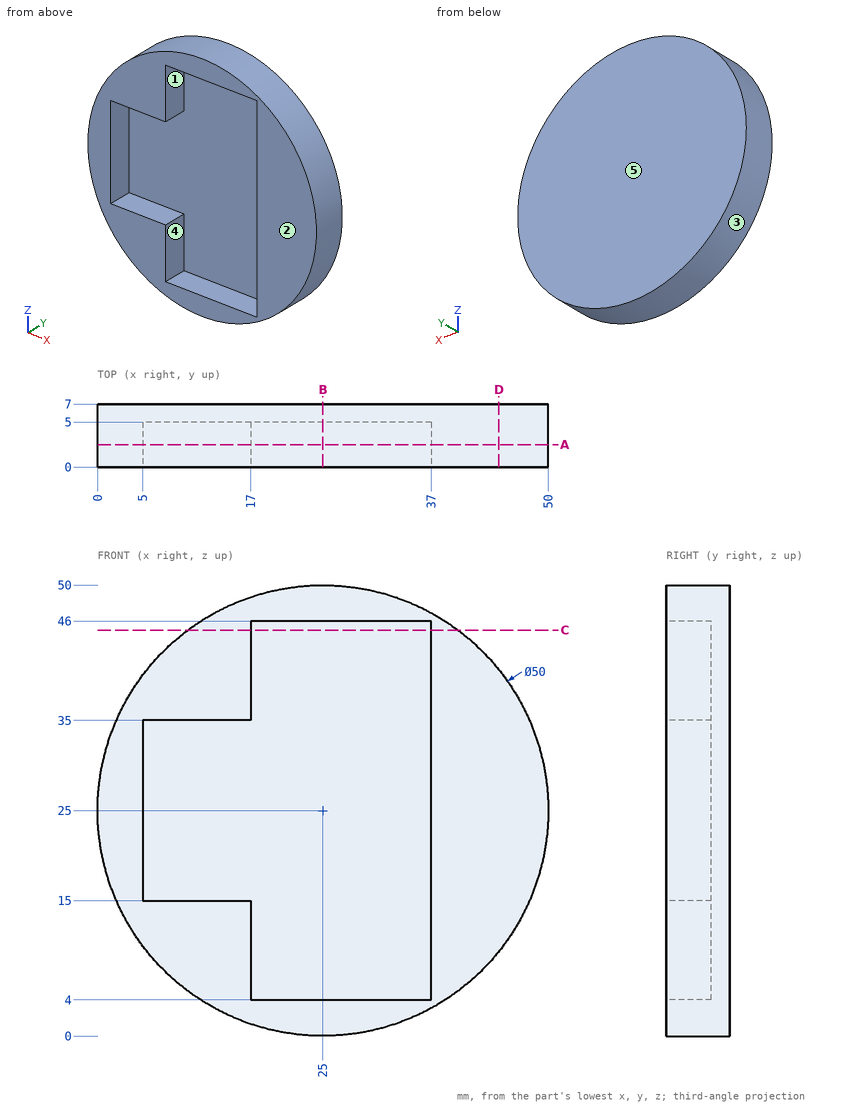
Here's the drawing with two shaded views (mm, measured from the low corner). I have some questions. A direction names the side the tool comes from. Give positions to 0.01 mm unless a question says otherwise; leave off trailing zeros. Order: outer loops, then holes, each group sorted by start corner. A loop starts at its lowest first (then second) coordinate and runs counter-clockwise, first axis right, second up. Notation, with made-up numbers: (-16.5, 11.5) - (37.5, 11.5) arc R16 cw to (37.5, 30.5) - close; hole circle Ø9 at (46, 17.5). An arc over 180 degrees is marked (long way). Write each question's results on one line, items separated by ' | '.
1) Suppose I cut it at D-D, the plane x = 44.5. Write out the boundary of the cut face in (y, z), then the cut area to 3 significant figures.
Final values:
outline: (0, 9.36) - (7, 9.36) - (7, 40.64) - (0, 40.64) - close | area: 219 mm^2
2) Suppose I cut it at C-C, the plane z = 45. Write out the boundary of the cut face in (x, y).
Final values:
outline: (10, 0) - (17, 0) - (17, 5) - (37, 5) - (37, 0) - (40, 0) - (40, 7) - (10, 7) - close
3) If we mould it in two halves opening along Z, with no side actions, what happens to the marked faces 3, 4 and 5? For each: pulls with the +Z half, pulls with the -Z half, needs draft (parallel to the pull), parting line crosses it, or undercut.
Final values:
face 3: parting line crosses it | face 4: undercut | face 5: needs draft
4) Please list where these lines run through material, in increasing order: line 1 along Y through (x, z) = (6.5, 30); line 2 along Z through (x, y) = (33.5, 1); line 3 along X through (y, z) = (3.25, 14). Write a range as [from, to].
Final values:
line 1: y = [5, 7] | line 2: z = [1.49, 4], [46, 48.51] | line 3: x = [2.55, 17], [37, 47.45]
5) I'm going to push flat-ended pins straight in: pin 1 Ø4 at (x, y) = (12, 2.5) entering from +Z; pin 2 Ø1.5 at (x, z) = (40.5, 14) entering from -Y; pin 3 Ø4 at (x, y) = (7.5, 5.5) entering from +Z; pin 4 Ø4 at (y, z) = (1.5, 15.5) entering from -X. Where does each tip first touch, or does it pass through?
Final values:
pin 1: stops at z = 47.45 | pin 2: stops at y = 0 | pin 3: stops at z = 44.62 | pin 4: stops at x = 1.15
6) On a 3-axis mill with a long thin cutter (end or side, diameter ignored), from which of +Z, -Z, +X, -X, +Y, -Y can I reach the whole of each face in a straight line? I mean the marked faces 1 and 2. Say none if no direction works.
Final values:
face 1: -Y | face 2: +Z, -Z, +X, -X, -Y
7) Suppose I cut it at B-B, the plane x = 25. Write out the boundary of the cut face in (y, z).
Final values:
outline: (0, 0) - (7, 0) - (7, 50) - (0, 50) - (0, 46) - (5, 46) - (5, 4) - (0, 4) - close
8) Suppose I cut it at A-A, the plane y = 2.5. Write out the boundary of the cut face in (x, z), then the cut area to 3 significant figures.
Final values:
outline: circle Ø50 at (25, 25); hole (5, 15) - (17, 15) - (17, 4) - (37, 4) - (37, 46) - (17, 46) - (17, 35) - (5, 35) - close | area: 883 mm^2
